from build123d import *

# Parameters (mm, degrees)
F0_W           = 76.0650336742
F0_H           = 65.9612175077
F1_DEPTH       = 38.354
F2_R           = 5.08
F4_D           = 5.5
F4_CBORE_D     = 9.75
F4_CBORE_DEPTH = 5


with BuildPart() as f1:
    # F0 (on Top) → F1 (new body)
    with BuildSketch(Plane.XY):
        with Locations((2.9734522104, 3.0732313171)):
            Rectangle(F0_W, F0_H)
    extrude(amount=F1_DEPTH)

    # F2
    f2_edges = [f1.edges().sort_by_distance(p)[0] for p in [
        (2.973452, -29.907377, 38.354),
        (41.005969, 3.073231, 38.354),
        (2.973452, 36.05384, 38.354),
        (-35.059065, 3.073231, 38.354),
    ]]
    fillet(f2_edges, radius=F2_R)

    # F4 (through all)
    with Locations(Plane.XY.offset(38.354)):
        with Locations((-13.5124307126, 5.8261519298), (19.4780696183, -11.7112351581)):
            CounterBoreHole(F4_D / 2, F4_CBORE_D / 2, F4_CBORE_DEPTH)


solid = f1.part
Design review of the part built by this model. Coordinates are the model's own, in mm. A direction names the side the tool comes from. Coordinates: 2 decimals unless noted, no trailing zeros. Write each loop counter-clockwise with the first axis right and the second up, starting at its lowest first coordinate (ties: lowest second). Pieces come first, ordered by that corner, then holes. Notation, with made-up numbers: (34.5, 66) - (86.5, 66) arc R21 ccw to (86.5, 74) - close; hole circle Ø8 at (52, 56.5). An arc over 180 degrees is marked (long way). Use one line per item in the form item = value.
Q1. For probe 1 along X at (y, z) = (-12, 17); probe 2 along X at (y, z) = (7.5, 14.5); probe 3 along Y at (x, z) = (-11.5, 16), list the stretches that pass through material, from the lowest coordinate up.
Taken from the geometry:
probe_1 = -35.06 to 16.74, 22.21 to 41.01
probe_2 = -35.06 to -15.69, -11.33 to 41.01
probe_3 = -29.91 to 3.95, 7.7 to 36.05
Q2. Insertion check: pin 1 Ø6.5 at (x, y) = (19.48, -11.71) entering from +Z. The pin has a flat end and moves straight along its axis. Give the tip position at first contact, or say it passes through.
Taken from the geometry:
pin_1 = 33.35
Q3. Consider section B-B (y = 4.5). Write out the cut boundary in (x, z), plus the area to 3 significant figures.
Taken from the geometry:
outline = (-35.06, 0) - (-15.92, 0) - (-15.92, 33.35) - (-18.2, 33.35) - (-18.2, 38.35) - (-29.98, 38.35) arc R5.08 ccw to (-35.06, 33.27) - close; (-11.1, 0) - (41.01, 0) - (41.01, 33.27) arc R5.08 ccw to (35.93, 38.35) - (-8.82, 38.35) - (-8.82, 33.35) - (-11.1, 33.35) - close
area = 2,700 mm^2
Q4. Machinability: for faces 1 (the flat face through (3, 3, 38.354)), 2 (the cylindrical face through (-9.01, 3.96, 35.89)), which of the approach directions +Z, -Z, +X, -X, +Y, -Y give a long, thin tool a straight path to every point of the face, cutting with its end or side? Answer none if there is none.
Taken from the geometry:
face_1 = +Z, +X, -X, +Y, -Y
face_2 = +Z
Q5. Consider section A-A (y = -10). Write out the cut boundary in (x, z), plus the area to 3 significant figures.
Taken from the geometry:
outline = (-35.06, 0) - (17.33, 0) - (17.33, 33.35) - (14.91, 33.35) - (14.91, 38.35) - (-29.98, 38.35) arc R5.08 ccw to (-35.06, 33.27) - close; (21.63, 0) - (41.01, 0) - (41.01, 33.27) arc R5.08 ccw to (35.93, 38.35) - (24.04, 38.35) - (24.04, 33.35) - (21.63, 33.35) - close
area = 2,720 mm^2
Q6. The part is to be moulded in two halves that separate along X. For faces 3 (the flat face through (2, -29.907, 16)), 4 (the flat face through (-35.059, 3, 16)), 5 (the cylindrical face through (16.855, -10.885, 16.444)), say which applies: +X half, -X half, draft (parallel to the pull), parting line (faces both ways), or undercut.
Taken from the geometry:
face_3 = draft
face_4 = -X half
face_5 = undercut
